from build123d import *

# Parameters (mm, degrees)
SKETCH2_R           = 40
BOSS_EXTRUDE1_DEPTH = 76
SKETCH3_W           = 8
SKETCH3_H           = 20
CUT_EXTRUDE1_DEPTH  = 3
SKETCH4_R           = 42
SKETCH4_R_2         = 40
BOSS_EXTRUDE3_DEPTH = 28
SKETCH5_W           = 56.5
SKETCH5_H           = 56.5
CUT_EXTRUDE7_DEPTH  = 5
SKETCH6_R           = 2
CUT_EXTRUDE8_DEPTH  = 93.568893263
SKETCH7_R           = 2.5
CUT_EXTRUDE9_DEPTH  = 97.457244414


with BuildPart() as part:
    # Sketch2 → Boss-Extrude1 (new body)
    with BuildSketch(Plane(origin=(0, 0, 0), x_dir=(1, 0, 0), z_dir=(0, 1, 0))):
        with Locations(Location((0, 0, 0), (0, 0, 270))):
            Circle(SKETCH2_R)
        with BuildLine():
            Line((-16.05, 28.2), (16.05, 28.2))
            ThreePointArc((16.05, 28.2), (18.171320344, 27.321320344), (19.05, 25.2))
            Line((19.05, 25.2), (19.05, 24.05))
            ThreePointArc((19.05, 24.05), (20.514466094, 20.514466094), (24.05, 19.05))
            Line((24.05, 19.05), (25.2, 19.05))
            ThreePointArc((25.2, 19.05), (27.321320344, 18.171320344), (28.2, 16.05))
            Line((28.2, 16.05), (28.2, -16.05))
            ThreePointArc((28.2, -16.05), (27.321320344, -18.171320344), (25.2, -19.05))
            Line((25.2, -19.05), (24.05, -19.05))
            ThreePointArc((24.05, -19.05), (20.514466094, -20.514466094), (19.05, -24.05))
            Line((19.05, -24.05), (19.05, -25.2))
            ThreePointArc((19.05, -25.2), (18.171320344, -27.321320344), (16.05, -28.2))
            Line((16.05, -28.2), (-16.05, -28.2))
            ThreePointArc((-16.05, -28.2), (-18.171320344, -27.321320344), (-19.05, -25.2))
            Line((-19.05, -25.2), (-19.05, -24.05))
            ThreePointArc((-19.05, -24.05), (-20.514466094, -20.514466094), (-24.05, -19.05))
            Line((-24.05, -19.05), (-25.2, -19.05))
            ThreePointArc((-25.2, -19.05), (-27.321320344, -18.171320344), (-28.2, -16.05))
            Line((-28.2, -16.05), (-28.2, 16.05))
            ThreePointArc((-28.2, 16.05), (-27.321320344, 18.171320344), (-25.2, 19.05))
            Line((-25.2, 19.05), (-24.05, 19.05))
            ThreePointArc((-24.05, 19.05), (-20.514466094, 20.514466094), (-19.05, 24.05))
            Line((-19.05, 24.05), (-19.05, 25.2))
            ThreePointArc((-19.05, 25.2), (-18.171320344, 27.321320344), (-16.05, 28.2))
        make_face(mode=Mode.SUBTRACT)
    extrude(amount=BOSS_EXTRUDE1_DEPTH)

    # Sketch3 → Cut-Extrude1 (cut)
    with BuildSketch(Plane(origin=(0, 0, 28.2), x_dir=(-1, 0, 0), z_dir=(0, 0, -1))):
        with Locations((0, 10)):
            Rectangle(SKETCH3_W, SKETCH3_H)
    extrude(amount=-CUT_EXTRUDE1_DEPTH, mode=Mode.SUBTRACT)

    # Sketch4 → Boss-Extrude3 (add, symmetric)
    with BuildSketch(Plane(origin=(0, 38, 0), x_dir=(1, 0, 0), z_dir=(0, 1, 0))):
        with Locations(Location((0, 0, 0), (0, 0, 270))):
            Circle(SKETCH4_R)
        with Locations(Location((0, 0, 0), (0, 0, 270))):
            Circle(SKETCH4_R_2, mode=Mode.SUBTRACT)
    extrude(amount=BOSS_EXTRUDE3_DEPTH, both=True)

    # Sketch5 → Cut-Extrude7 (cut)
    with BuildSketch(Plane(origin=(0, 76, 0), x_dir=(1, 0, 0), z_dir=(0, 1, 0))):
        Rectangle(SKETCH5_W, SKETCH5_H)
    extrude(amount=-CUT_EXTRUDE7_DEPTH, mode=Mode.SUBTRACT)

    # Sketch6 → Cut-Extrude8 (cut, through all)
    with BuildSketch(Plane(origin=(0, 71, 0), x_dir=(1, 0, 0), z_dir=(0, 1, 0))):
        with Locations(Location((-23.55, 23.55, 0), (0, 0, 270))):
            Circle(SKETCH6_R)
        with Locations(Location((23.55, 23.55, 0), (0, 0, 270))):
            Circle(SKETCH6_R)
        with Locations(Location((23.55, -23.55, 0), (0, 0, 270))):
            Circle(SKETCH6_R)
        with Locations(Location((-23.55, -23.55, 0), (0, 0, 270))):
            Circle(SKETCH6_R)
    extrude(amount=-CUT_EXTRUDE8_DEPTH, mode=Mode.SUBTRACT)

    # Sketch7 → Cut-Extrude9 (cut, through all)
    with BuildSketch(Plane(origin=(0, 76, 0), x_dir=(1, 0, 0), z_dir=(0, 1, 0))):
        with Locations(Location((0, 35, 0), (0, 0, 270))):
            Circle(SKETCH7_R)
        with Locations(Location((35, 0, 0), (0, 0, 270))):
            Circle(SKETCH7_R)
        with Locations(Location((0, -35, 0), (0, 0, 270))):
            Circle(SKETCH7_R)
        with Locations(Location((-35, 0, 0), (0, 0, 270))):
            Circle(SKETCH7_R)
    extrude(amount=-CUT_EXTRUDE9_DEPTH, mode=Mode.SUBTRACT)


solid = part.part
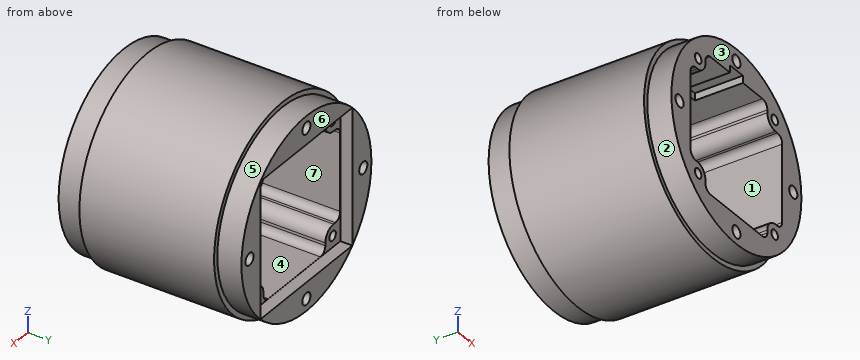
Geometry: final body of the model. Coordinates: model frame, mm. Face numbers are marked on the shaded views. A direction names the side the tool comes from. Give positions to 0.01 mm unless a question says otherwise; leave off trailing zeros. Write each loop counter-clockwise with the first axis right and the second up, starting at its lowest first coordinate (ties: lowest second). Pieces come first, ordered by that corner, then holes. Notation, with made-up numbers: (58.5, 34) -> (74.5, 34) arc R21 ccw to (74.5, 39) -> close; hole circle Ø10 at (85.5, 84). An arc over 180 degrees is marked (long way). Answer as a JSON object with one key per item and string values.
1. Ray query, probe 1 along X at (y, z) = (40.5, -24.5); probe 2 along X at (y, z) = (19, 23.55). Return the intervals inside material, ascending. Write a range as from..to.
Ans:
{"probe 1": "x = -34.11..-25.31, -21.79..-19.05, 19.05..21.79, 25.31..34.11", "probe 2": "x = -34.78..-25.55, -21.55..-19.08, 19.08..21.55, 25.55..34.78"}
2. Cut plane A-A on y = 56.5. Count the separate pieces of the cut face and the enclosed holes in it, and give its area (3 significant figures).
Ans:
{"separate pieces": "1", "enclosed holes": "9", "area": "2,560 mm^2"}
3. Cut plane B-B on z = 12.5. Output: boundary loops of the cut face in (x, y), and give its area (3 significant figures).
Ans:
{"outline": "(-40.1, 10) -> (-38, 10) -> (-38, 0) -> (-28.2, 0) -> (-28.2, 71) -> (-28.25, 71) -> (-28.25, 76) -> (-38, 76) -> (-38, 66) -> (-40.1, 66) -> close; (28.2, 0) -> (38, 0) -> (38, 10) -> (40.1, 10) -> (40.1, 66) -> (38, 66) -> (38, 76) -> (28.25, 76) -> (28.25, 71) -> (28.2, 71) -> close", "area": "1,720 mm^2"}
4. Contact query for flat-ended pins moving along their axis: pin 1 (2 mm diameter, centred on x = 2, y = 34.5, fed in from +Z); pin 2 (1 mm diameter, centred on x = 7, y = 17.5, fed in from +Z); pin 3 (16 mm diameter, centred on y = 44, z = 0, fed in from -X). Output: stop coordinate, or through.
Ans:
{"pin 1": "stops at z = 41.99", "pin 2": "stops at z = 41.49", "pin 3": "stops at x = -42"}
5. Access query for the marked faces 1, 2 and 3. Directions: +Z, -Z, +X, -X, +Y, -Y. A direction counts if a zero-diameter tool reaches every point of the face in a straight line with its end or side. Return the directions, or none.
Ans:
{"face 1": "+Y, -Y", "face 2": "-Y", "face 3": "+Z, -Z, +X, -X, -Y"}
6. Cut plane C-C on x = 35. Output: boundary loops of the cut face in (y, z).
Ans:
{"outline": "(0, -19.36) -> (10, -19.36) -> (10, -23.22) -> (66, -23.22) -> (66, -19.36) -> (76, -19.36) -> (76, -2.5) -> (0, -2.5) -> close; (0, 2.5) -> (76, 2.5) -> (76, 19.36) -> (66, 19.36) -> (66, 23.22) -> (10, 23.22) -> (10, 19.36) -> (0, 19.36) -> close"}
7. Cut plane D-D on z = -34. Output: boundary loops of the cut face in (x, y).
Ans:
{"outline": "(-24.66, 10) -> (-21.07, 10) -> (-21.07, 0) -> (-2.29, 0) -> (-2.29, 76) -> (-21.07, 76) -> (-21.07, 66) -> (-24.66, 66) -> close; (2.29, 0) -> (21.07, 0) -> (21.07, 10) -> (24.66, 10) -> (24.66, 66) -> (21.07, 66) -> (21.07, 76) -> (2.29, 76) -> close"}
8. Mould query, pull axis Z, two halves, no side actions, for the marked faces 4, 5, 6 and 7. Classes: pulls with the +Z half, pulls with the -Z half, needs draft (parallel to the pull), parting line crosses it, or undercut.
Ans:
{"face 4": "undercut", "face 5": "parting line crosses it", "face 6": "needs draft", "face 7": "undercut"}
